For this review, take the finished solid that the model builds, in its own axes (mm). Face numbers are marked on the shaded views. A direction names the side the tool comes from. Coordinates: 2 decimals unless noted, no trailing zeros. Order: outer loops, then holes, each group sorted by start corner. A loop starts at its lowest first (then second) coordinate and runs counter-clockwise, first axis right, second up. Notation, with made-up numbers: (41.5, 32.25) -> (59.5, 32.25) arc R17 ccw to (59.5, 43.25) -> close; hole circle Ø6 at (89, 19). An arc over 180 degrees is marked (long way). Return JSON: item names as keys, results as strings. Group by question number.
Item 1: Take a section at D-D (y = 0). Write out the cut boundary in (x, z).
Item 2: Draft analysis for pull direction Y (two halves, no side actions). For the marked faces 1, 2, 3 and 4, state which applies: +Y half, -Y half, draft (parallel to the pull), parting line (faces both ways), or undercut.
Item 3: For line 1 along X through (y, z) = (-17.5, 102); line 2 along Y through (x, z) = (15, 91.5); line 3 along Y through (x, z) = (23.5, 148), list the stretches that pass through material, from the lowest coordinate up.
Item 4: Machinability: for the marked faces 5 and 6, which of the approach directions +Z, -Z, +X, -X, +Y, -Y give a long, thin tool a straight path to every point of the face, cutting with its end or side? Answer none if there is none.
Item 5: Take a section at A-A (z = 41.5). Write out the cut boundary in (x, y), then the cut area to 3 significant figures.
Item 6: Insertion check: pin 1 (6 mm diameter, centred on x = 11.5, y = -26, fed in from +Z); pin 2 (11 mm diameter, centred on y = -1, z = 72.5, fed in from +X); pin 3 (8 mm diameter, centred on y = -19.5, z = 70.5, fed in from +X). Each pin has a flat end and moves straight along its axis. Give the tip position at first contact, or say it passes through.
Autodesk Inventor part; units mm, degrees
ref_plane "Начальная плоскость" through (0, 0, -26.9242) normal (0, 0, 1) x (1, 0, 0)
ref_plane "Конечная плоскость" through (0, 0, 247.3386) normal (0, 0, 1) x (1, 0, 0)
ref_plane "РабПлоскость8" through (-29, 196.7514, 385.3079) normal (0, -0.6432, 0.7657) x (1, 0, 0)
ref_plane "Начальная плоскость" through (0, 0, -26.9242) normal (0, 0, 1) x (1, 0, 0)
ref_plane "Конечная плоскость" through (0, 0, 247.3386) normal (0, 0, 1) x (1, 0, 0)
sketch "Эскиз" plane through (0, 0, 0) normal (0, 0, 1) x (1, 0, 0)
  line L0 (36, -32.5) -> (0, -32.5)
  line L1 (36, -32.5) -> (36, -28.696)
  line L2 (33.6994, -26.2039) -> (9.9215, -24.3017)
  line L3 (4.4, -18.3208) -> (4.4, 18.3208)
  line L4 (33.6994, 26.2039) -> (9.9215, 24.3017)
  line L5 (36, 28.696) -> (36, 32.5)
  line L6 (0, 32.5) -> (36, 32.5)
  line L7 (0, -32.5) -> (0, 32.5)
  arc A0 (4.4, -18.3208) -> (9.9215, -24.3017) centre (10.4, -18.3208) ccw
  arc A1 (9.9215, 24.3017) -> (4.4, 18.3208) centre (10.4, 18.3208) ccw
  arc A2 (36, -28.696) -> (33.6994, -26.2039) centre (33.5, -28.696) ccw
  arc A3 (33.6994, 26.2039) -> (36, 28.696) centre (33.5, 28.696) ccw
  line L8 (0, 45.5) -> (0, -45.5) construction
  line L9 (-7.2974, 0) -> (43.7847, 0) construction
  point P0 (36, -26.388)
  point P1 (4.4, -23.86)
  point P2 (4.4, 23.86)
  point P3 (36, 26.388)
  dimension "d3" = 36
  dimension "d5" = 4.4
  dimension "d7" = 65
  dimension "d9" = 8.64
  dimension "d11" = 8.64
  dimension "d13" = 6.112
  dimension "d15" = 6.112
  dimension "d22" = 6
  dimension "d23" = 2.5
  dimension "d24" = 32.5
  dimension "d25" = 0
extrude "Тело" add sketch "Эскиз" along normal up to surface (274.2628 mm away) from surface at -26.9242
sketch "Sketch3" plane through (0, 0, 0) normal (0, 0, 1) x (1, 0, 0)
  line L0 (0, 0) -> (10, 0)
ref_plane "Work Plane7" through (0, 0, 0) normal (0, -1, 0) x (1, 0, 0)
sketch "Sketch4" plane through (0, 0, 0) normal (0, -1, 0) x (1, 0, 0)
  line L0 (-2, -26.9242) -> (12, -26.9242)
  line L1 (-2, 247.3386) -> (12, 247.3386)
  dimension "d29" = 274.2629
ref_plane "РабПлоскость8" through (-29, 196.7514, 385.3079) normal (0, -0.6432, 0.7657) x (1, 0, 0)
split "Разделение1" plane through (-29, 196.7514, 385.3079) removes the side toward (0, -0.6432, 0.7657)
ref_plane "РабПлоскость9" through (36, 522.1937, 436.4622) normal (0, 0.6411, -0.7674) x (1, 0, 0)
split "Разделение2" plane through (36, 522.1937, 436.4622) removes the side toward (0, 0.6411, -0.7674)
equation "\"d3\" = b"
equation "\"d7\" = ParH"
equation "\"d22\" = R"
equation "\"d23\" = R1"
equation "\"d24\" = 0.5 * d7"
equation "\"d16\" = G_L"
equation "\"R1\" = 2.5"
equation "\"R\" = 6"
equation "\"t1\" = 4.4"
equation "\"t2\" = 7.2"
equation "\"ParH\" = 65"
equation "\"b\" = 36"
equation "\"msp_x1\" = 0.04 * b"
equation "\"msp_x2\" = -0.08 * t1 + 0.04 * b"
equation "\"G_L\" = d29"
equation "\"ex\" = 0"
equation "\"G_OFFSET_START\" = 26.92422"
equation "\"G_OFFSET_END\" = 27.29963"
equation "\"d26\" = -G_OFFSET_START"
equation "\"d27\" = G_OFFSET_END + B_L"
equation "\"B_L\" = 220.039"
properties part number "Швеллер 6.5U-274,26 ГОСТ 8240-97" material "Сталь, мягкая"
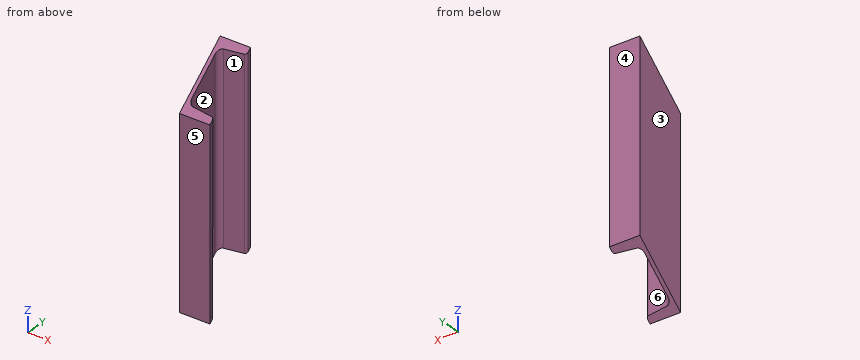
Findings below:
{
 "1": {"outline": "(0, 0.21) -> (4.4, 0.21) -> (4.4, 220.03) -> (0, 220.03) -> close"},
 "2": {"face 1": "undercut", "face 2": "undercut", "face 3": "draft", "face 4": "+Y half"},
 "3": {"line 1": "x = 0 to 4.4", "line 2": "y = -32.5 to -24.71, 24.71 to 32.5", "line 3": "y = -32.5 to -25.39, 25.39 to 32.5"},
 "4": {"face 5": "+Z, -Z, +X, -X, -Y", "face 6": "+Z, -Z, +X"},
 "5": {"outline": "(0, -32.5) -> (36, -32.5) -> (36, -28.7) arc R2.5 ccw to (33.7, -26.2) -> (9.92, -24.3) arc R6 cw to (4.4, -18.32) -> (4.4, 18.32) arc R6 cw to (9.92, 24.3) -> (33.7, 26.2) arc R2.5 ccw to (36, 28.7) -> (36, 32.5) -> (0, 32.5) -> close", "area": "763 mm2"},
 "6": {"pin 1": "stops at z = 199.72", "pin 2": "stops at x = 4.4", "pin 3": "stops at x = 7.37"}
}
